The drawing under review shows one solid part. Ordinate dimensions are in mm from its lowest x, y, z. Round coordinates to 2 decimals unless told otherwise and drop trailing zeros. Loops run counter-clockwise (first coordinate to the right, second up) from the corner with the lowest first, then second, coordinate; pieces in that order, holes last. Notation, with made-up numbers: (59, 32.5) - (110, 32.5) arc R14 cw to (110, 53.5) - close; hole circle Ø1 at (-21, 39.25). An arc over 180 degrees is marked (long way). Answer as CSV lines item,"result".
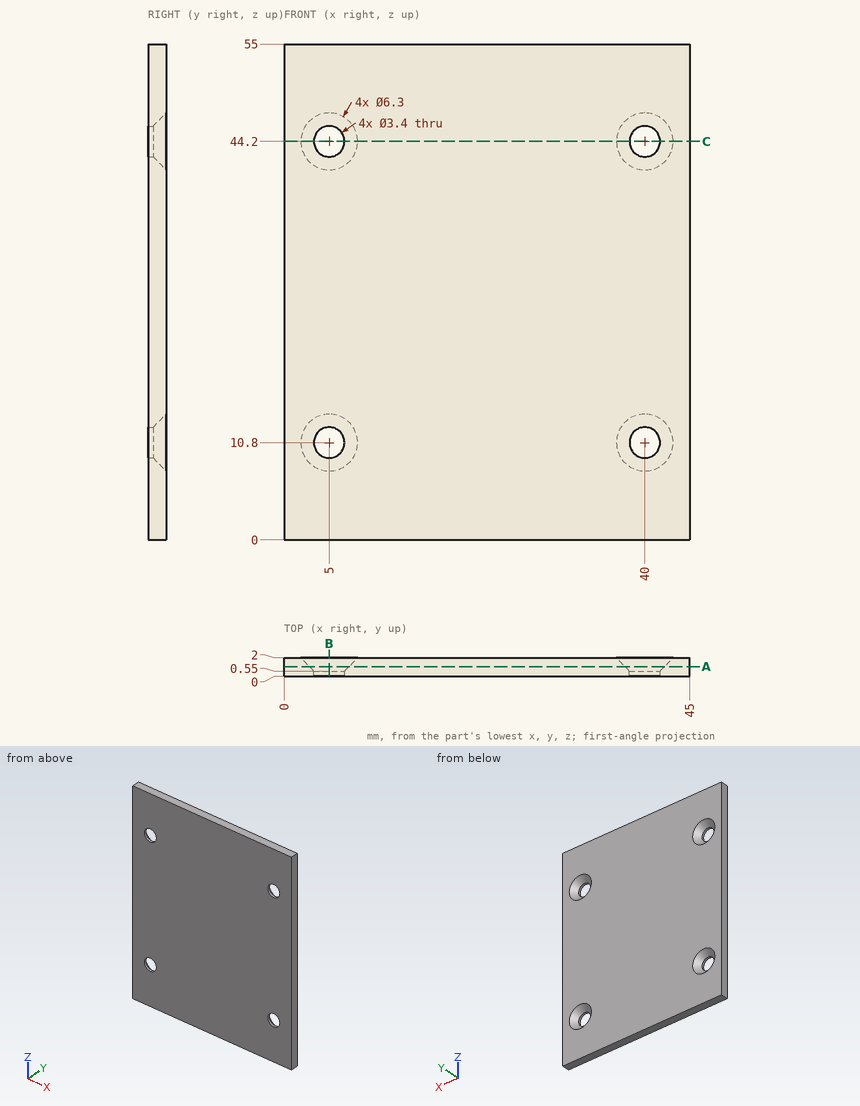
1. Take a section at A-A (y = 1.05). State the section outline as (x, z) points, plus the area to 3 significant figures.
Numbers:
outline,"(0, 0) - (45, 0) - (45, 55) - (0, 55) - close; hole circle Ø4.4 at (5, 10.8); hole circle Ø4.4 at (5, 44.2); hole circle Ø4.4 at (40, 10.8); hole circle Ø4.4 at (40, 44.2)"
area,"2,410 mm²"
2. Take a section at C-C (z = 44.2). State the section outline as (x, y) points.
Numbers:
outline,"(0, 0) - (3.3, 0) - (3.3, 0.55) - (1.85, 2) - (0, 2) - close; (6.7, 0) - (38.3, 0) - (38.3, 0.55) - (36.85, 2) - (8.15, 2) - (6.7, 0.55) - close; (41.7, 0) - (45, 0) - (45, 2) - (43.15, 2) - (41.7, 0.55) - close"
3. Take a section at B-B (x = 5). State the section outline as (y, z) points, plus the area to 3 significant figures.
Numbers:
outline,"(0, 0) - (2, 0) - (2, 7.65) - (0.55, 9.1) - (0, 9.1) - close; (0, 12.5) - (0.55, 12.5) - (2, 13.95) - (2, 41.05) - (0.55, 42.5) - (0, 42.5) - close; (0, 45.9) - (0.55, 45.9) - (2, 47.35) - (2, 55) - (0, 55) - close"
area,"92.2 mm²"
4. Clearance check with flat-ended pins moving along their axes: pin 1 (4 mm diameter, centred on x = 5, z = 44.2, fed in from +Y); pin 2 (6 mm diameter, centred on x = 21, z = 32.5, fed in from -Y). State where each tip first meets the part, or that it passes through.
Numbers:
pin 1,"stops at y = 0.85"
pin 2,"stops at y = 0"
5. Wall thickness on probe 1 along X at (y, z) = (0.3, 44.2); probe 2 along Z at (x, y) = (40, 0.3); probe 3 along X at (y, z) = (0.8, 45): over which ranges is each line inside the solid? List them lowest first.
Numbers:
probe 1,"x = 0 to 3.3, 6.7 to 38.3, 41.7 to 45"
probe 2,"z = 0 to 9.1, 12.5 to 42.5, 45.9 to 55"
probe 3,"x = 0 to 3.22, 6.78 to 38.22, 41.78 to 45"
